Verification items for the finished model (mm, model axes). Face numbers are marked on the shaded views. A direction names the side the tool comes from. Coordinates: 2 decimals unless noted, no trailing zeros. Order: outer loops, then holes, each group sorted by start corner. A loop starts at its lowest first (then second) coordinate and runs counter-clockwise, first axis right, second up. Notation, with made-up numbers: (-33, -22.75) -> (-11, -22.75) arc R27 ccw to (-11, 16.25) -> close; hole circle Ø9 at (13.5, 67). An arc over 180 degrees is marked (long way). Answer as CSV lines item,"result".
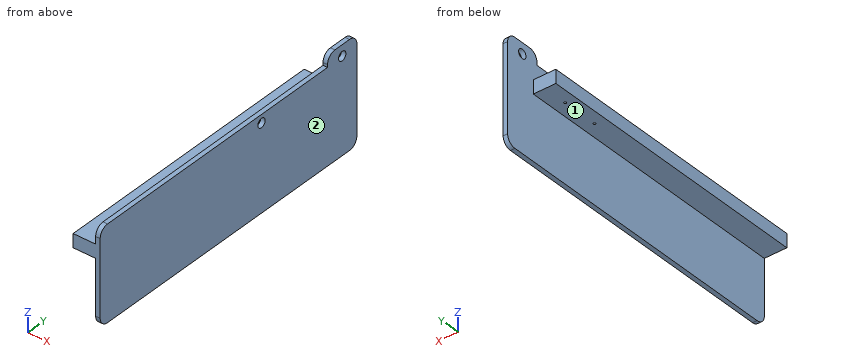
```python
from build123d import *

# Parameters (mm, degrees)
F0_R     = 5
F1_DEPTH = 5
F2_W     = 315
F2_H     = 15
F3_DEPTH = 25
F5_D     = 2.6


with BuildPart() as f1:
    # F0 (on Right) → F1 (new body)
    with BuildSketch(Plane.YZ):
        with BuildLine():
            Line((-20, -1), (-320, -1))
            ThreePointArc((-320, -1), (-327.071068, -3.928932), (-330, -11))
            Line((-330, -11), (-330, -95))
            ThreePointArc((-330, -95), (-327.071068, -102.071068), (-320, -105))
            Line((-320, -105), (10, -105))
            ThreePointArc((10, -105), (17.071068, -102.071068), (20, -95))
            Line((20, -95), (20, 2))
            ThreePointArc((20, 2), (17.071068, 9.071068), (10, 12))
            Line((10, 12), (-10, 12))
            ThreePointArc((-10, 12), (-17.071068, 9.071068), (-20, 2))
            Line((-20, 2), (-20, -1))
        make_face()
        with Locations((-110, -10)):
            Circle(F0_R, mode=Mode.SUBTRACT)
        Circle(F0_R, mode=Mode.SUBTRACT)
    extrude(amount=F1_DEPTH)

    # F2 (on face) → F3 (join)
    with BuildSketch(Plane(origin=(0, 0, 0), x_dir=(0, -1, 0), z_dir=(-1, 0, 0))):
        with Locations((172.5, -26.5)):
            Rectangle(F2_W, F2_H)
    extrude(amount=F3_DEPTH)

    # F5 (through all)
    with Locations(Plane.XY.offset(-19)):
        with Locations((-13, -42.403466), (-13, -82.403466)):
            Hole(F5_D / 2)


solid = f1.part
```
Item 1: Depth check by flat-ended pin: pin 1 Ø2.5 at (x, y) = (-13, -82.4) entering from +Z; pin 2 Ø12.5 at (x, y) = (-9, -157.5) entering from -Z; pin 3 Ø10 at (y, z) = (-283.5, -90.5) entering from -X; pin 4 Ø2.5 at (x, z) = (3.5, 0.5) entering from -Y. Enter the tip coordinate at first touch or a pass-through.
Answer list:
pin 1,"through"
pin 2,"z = -34"
pin 3,"x = 0"
pin 4,"y = -20"
Item 2: Section check D-D, the plane y = -66. Record the boundary of the cut face in (x, z), plus the area to 3 significant figures.
Answer list:
outline,"(-25, -34) -> (0, -34) -> (0, -105) -> (5, -105) -> (5, -1) -> (0, -1) -> (0, -19) -> (-25, -19) -> close"
area,"895 mm2"
Item 3: Section check C-C, the plane x = -18.5. Record the boundary of the cut face in (y, z).
Answer list:
outline,"(-330, -34) -> (-15, -34) -> (-15, -19) -> (-330, -19) -> close"
Item 4: Section check A-A, the plane y = 0. Record the boundary of the cut face in (x, z), plus the area to 3 significant figures.
Answer list:
outline,"(0, -105) -> (5, -105) -> (5, -5) -> (0, -5) -> close; (0, 5) -> (5, 5) -> (5, 12) -> (0, 12) -> close"
area,"535 mm2"
Item 5: Section check B-B, the plane y = -110. Record the boundary of the cut face in (x, z), plus the area to 3 significant figures.
Answer list:
outline,"(-25, -34) -> (0, -34) -> (0, -105) -> (5, -105) -> (5, -15) -> (0, -15) -> (0, -19) -> (-25, -19) -> close; (0, -5) -> (5, -5) -> (5, -1) -> (0, -1) -> close"
area,"845 mm2"
Item 6: Thickness scan on line 1 (Z direction, x = 2.55, y = -110); line 2 (Z direction, x = 3.05, y = 0); line 3 (Z direction, x = -5.25, y = -17). Record the ranges inside material, lowest first.
Answer list:
line 1,"-105 to -15, -5 to -1"
line 2,"-105 to -5, 5 to 12"
line 3,"-34 to -19"
Item 7: Tool access check on the marked faces 1 and 2. Record the directions out of +Z, -Z, +X, -X, +Y, -Y that give a thin tool (end or side, any length) a straight path to the whole face; none if there is none.
Answer list:
face 1,"-Z, -X, +Y, -Y"
face 2,"+Z, -Z, +X, +Y, -Y"
